```python
from build123d import *

# Parameters (mm, degrees)
SKETCH1_W           = 160
SKETCH1_H           = 28.575
BOSS_EXTRUDE1_DEPTH = 28.575
SKETCH3_W           = 147.3
SKETCH3_H           = 28.575
CUT_EXTRUDE3_DEPTH  = 19.05
SKETCH4_W           = 76.2
SKETCH4_H           = 8
BOSS_EXTRUDE2_DEPTH = 45.4
CUT_EXTRUDE8_DEPTH  = 124.871382326
SKETCH9_R           = 4.7625
BOSS_EXTRUDE4_DEPTH = 12.525
SKETCH10_R          = 4.7625
CUT_EXTRUDE10_DEPTH = 124.871382326
CUT_EXTRUDE11_START = -41.9
SKETCH2_OUTSIDE_W   = 111.689
SKETCH2_OUTSIDE_H   = 66.289
SKETCH2_OUTSIDE_R   = 14.2875
CUT_EXTRUDE11_DEPTH = 41.9
CUT_EXTRUDE13_START = -41.9
SKETCH13_OUTSIDE_W  = 111.689
SKETCH13_OUTSIDE_H  = 66.289
SKETCH13_OUTSIDE_R  = 14.2875
CUT_EXTRUDE13_DEPTH = 41.9
SKETCH14_R          = 11.1125
CUT_EXTRUDE14_DEPTH = 6.35
CUT_EXTRUDE15_START = -6.35
SKETCH15_R          = 11.1125
CUT_EXTRUDE15_DEPTH = 6.35


with BuildPart() as part:
    # Sketch1 → Boss-Extrude1 (new body)
    with BuildSketch(Plane(origin=(0, 0, 0), x_dir=(1, 0, 0), z_dir=(0, 1, 0))):
        with Locations((-20.782379652, -9.554800327)):
            Rectangle(SKETCH1_W, SKETCH1_H)
    extrude(amount=BOSS_EXTRUDE1_DEPTH)

    # Sketch3 → Cut-Extrude3 (cut)
    with BuildSketch(Plane(origin=(0, 28.575, 0), x_dir=(1, 0, 0), z_dir=(0, 1, 0))):
        with Locations((-20.782379652, -9.554800327)):
            Rectangle(SKETCH3_W, SKETCH3_H)
    extrude(amount=-CUT_EXTRUDE3_DEPTH, mode=Mode.SUBTRACT)

    # Sketch4 → Boss-Extrude2 (add)
    with BuildSketch(Plane.XY.offset(23.842300327)):
        with Locations((-20.782379652, 4.7625)):
            Rectangle(SKETCH4_W, SKETCH4_H)
    extrude(amount=BOSS_EXTRUDE2_DEPTH)

    # Sketch5 → Cut-Extrude8 (cut, through all)
    with BuildSketch(Plane(origin=(0, 8.7625, 0), x_dir=(1, 0, 0), z_dir=(0, 1, 0))):
        Polygon((-13.013921372, -46.075787503), (-13.013921372, -69.242300327), (17.317620348, -69.242300327), (17.317620348, -23.842300327), align=None)
        Polygon((-28.550837933, -69.242300327), (-28.550837933, -46.075787503), (-58.882379652, -23.842300327), (-58.882379652, -69.242300327), align=None)
    extrude(amount=-CUT_EXTRUDE8_DEPTH, mode=Mode.SUBTRACT)

    # Sketch9 → Boss-Extrude4 (add)
    with BuildSketch(Plane(origin=(0, 8.7625, 0), x_dir=(1, 0, 0), z_dir=(0, 1, 0))):
        with BuildLine():
            Line((-28.550837933, -46.075787503), (-28.550837933, -69.242300327))
            Line((-28.550837933, -69.242300327), (-13.013921372, -69.242300327))
            Line((-13.013921372, -69.242300327), (-13.013921372, -46.075787503))
            ThreePointArc((-13.013921372, -46.075787503), (-20.782379652, -32.954800327), (-28.550837933, -46.075787503))
        make_face()
        with Locations(Location((-20.782379652, -41.815004419, 0), (0, 0, 180))):
            Circle(SKETCH9_R, mode=Mode.SUBTRACT)
    extrude(amount=BOSS_EXTRUDE4_DEPTH)

    # Sketch10 → Cut-Extrude10 (cut, through all)
    with BuildSketch(Plane(origin=(0, 8.7625, 0), x_dir=(1, 0, 0), z_dir=(0, 1, 0))):
        with Locations(Location((-20.782379652, -41.815004419, 0), (0, 0, 180))):
            Circle(SKETCH10_R)
    extrude(amount=-CUT_EXTRUDE10_DEPTH, mode=Mode.SUBTRACT)

    # Sketch2 outside → Cut-Extrude11 (cut)
    with BuildSketch(Plane(origin=(59.217620348, 0, 0), x_dir=(0, 0, -1), z_dir=(1, 0, 0)).offset(CUT_EXTRUDE11_START)):
        with Locations((-32.2545, 14.2875)):
            Rectangle(SKETCH2_OUTSIDE_W, SKETCH2_OUTSIDE_H)
        with Locations((-9.554800327, 14.2875)):
            Circle(SKETCH2_OUTSIDE_R, mode=Mode.SUBTRACT)
    extrude(amount=CUT_EXTRUDE11_DEPTH, mode=Mode.SUBTRACT)

    # Sketch13 outside → Cut-Extrude13 (cut)
    with BuildSketch(Plane.ZY.offset(100.782379652).offset(CUT_EXTRUDE13_START)):
        with Locations((32.2545, 14.2875)):
            Rectangle(SKETCH13_OUTSIDE_W, SKETCH13_OUTSIDE_H)
        with Locations(Location((9.554800327, 14.2875, 0), (0, 0, 180))):
            Circle(SKETCH13_OUTSIDE_R, mode=Mode.SUBTRACT)
    extrude(amount=CUT_EXTRUDE13_DEPTH, mode=Mode.SUBTRACT)

    # Sketch14 → Cut-Extrude14 (cut)
    with BuildSketch(Plane(origin=(59.217620348, 0, 0), x_dir=(0, 0, -1), z_dir=(1, 0, 0))):
        with Locations((-9.554800327, 14.2875)):
            Circle(SKETCH14_R)
    extrude(amount=-CUT_EXTRUDE14_DEPTH, mode=Mode.SUBTRACT)

    # Sketch15 → Cut-Extrude15 (cut)
    with BuildSketch(Plane.ZY.offset(100.782379652).offset(CUT_EXTRUDE15_START)):
        with Locations(Location((9.554800327, 14.2875, 0), (0, 0, 180))):
            Circle(SKETCH15_R)
    extrude(amount=CUT_EXTRUDE15_DEPTH, mode=Mode.SUBTRACT)


solid = part.part
```
Here's how the part is built. I have some questions about the finished solid (model axes, mm). A direction names the side the tool comes from. Give positions to 0.01 mm unless a question says otherwise; leave off trailing zeros. Order: outer loops, then holes, each group sorted by start corner. A loop starts at its lowest first (then second) coordinate and runs counter-clockwise, first axis right, second up. Notation, with made-up numbers: M -12,-13.75 L 40,-13.75 A13 cw 40,-6.75 Z; hole C -31.5,73.25 d10. An arc over 180 degrees is marked long. Use a Markdown table: item, result. Add a question column.
1. Suppose I cut it at C-C (z = 15). List the corners of the cut face in (x, y) for me (3 decimals), and give its area (3 significant figures).
2. Suppose I cut it at D-D (y = 23.75). List the corners of the cut face in (x, z) for me.
3. Suppose I cut it at A-A (y = 16.25). List the corners of the cut face in (x, z) for me (1 decimal), and give its area (3 significant figures).
4. If we mould it in two halves opening along Y, with no side actions, what happens to faces 5 (the flat face through (-21, 21.288, 51)), 6 (the flat face through (-94.432, 7, 10)), 7 (the flat face through (-21, 0.763, 35)), 8 (the flat face through (-43.504, 4.818, 35.115))? For each: +Y half, -Y half, draft (parallel to the pull), parting line (faces both ways), or undercut.
5. For pin 1 Ø8 at (y, z) = (8, 6.5) entering from -X; pin 2 Ø8 at (y, z) = (7, 24.5) entering from +X; pin 3 Ø11 at (x, z) = (-34.5, 34) entering from +Y; pin 4 Ø14.5 at (x, z) = (-6.5, 8) entering from +Y (3 decimals), each with a flat end and sliding along its axis, tell me the tip position at first contact or that it passes through.
6. On a 3-axis mill with a long thin cutter (end or side, diameter ignored), from which of +Z, -Z, +X, -X, +Y, -Y can I reach the whole of each face in a straight line? I mean faces 1 (the cylindrical face through (-97.563, 10.95, -1.045)), 2 (the flat face through (-13.014, 11, 58)), 3 (the cylindrical face through (-20.53, 14.94, 32.96)), 4 (the flat face through (17.318, 3, -1)). Say none if no direction works.
7. I need wall thicknesses on probe 1 along X at (y, z) = (16, 42); probe 2 along X at (y, z) = (14.5, 54.5); probe 3 along X at (y, z) = (8.25, 13). Which ranges of each line are inside material? Lowest first, please. Write a range as from..to.
8. Suppose I cut it at B-B (x = -22.5). List the corners of the cut face in (y, z) for me (1 decimal), and give its area (3 significant figures).
Results list:
| question | item | result |
|---|---|---|
| 1 | outline | M -100.782,1.078 L -58.882,1.078 L -58.882,0 L 17.318,0 L 17.318,1.078 L 59.218,1.078 L 59.218,4.601 L 52.868,4.601 L 52.868,9.525 L -94.432,9.525 L -94.432,4.601 L -100.782,4.601 Z; M -100.782,23.974 L -94.432,23.974 L -94.432,27.497 L -100.782,27.497 Z; M 52.868,23.974 L 59.218,23.974 L 59.218,27.497 L 52.868,27.497 Z |
| 1 | area | 1,420 mm² |
| 2 | outline | M -100.78,-1.15 L -94.43,-1.15 L -94.43,3.73 L -100.78,3.73 Z; M -100.78,15.38 L -94.43,15.38 L -94.43,20.26 L -100.78,20.26 Z; M 52.87,-1.15 L 59.22,-1.15 L 59.22,3.73 L 52.87,3.73 Z; M 52.87,15.38 L 59.22,15.38 L 59.22,20.26 L 52.87,20.26 Z |
| 3 | outline | M -100.8,-4.6 L -94.4,-4.6 L -94.4,-1.4 L -100.8,-1.4 Z; M -100.8,20.5 L -94.4,20.5 L -94.4,23.7 L -100.8,23.7 Z; M -28.6,46.1 A8.9 ccw long -13,46.1 L -13,69.2 L -28.6,69.2 Z; M 52.9,-4.6 L 59.2,-4.6 L 59.2,-1.4 L 52.9,-1.4 Z; M 52.9,20.5 L 59.2,20.5 L 59.2,23.7 L 52.9,23.7 Z; hole C -20.8,41.8 d9.5 |
| 3 | area | 566 mm² |
| 4 | face 5 | +Y half |
| 4 | face 6 | undercut |
| 4 | face 7 | -Y half |
| 4 | face 8 | draft |
| 5 | pin 1 | stops at x = -94.43 |
| 5 | pin 2 | stops at x = 59.22 |
| 5 | pin 3 | stops at y = 8.76 |
| 5 | pin 4 | stops at y = 9.525 |
| 6 | face 1 | -X |
| 6 | face 2 | +Z, +X, +Y, -Y |
| 6 | face 3 | +Y |
| 6 | face 4 | -Z, +X, -Y |
| 7 | probe 1 | x = -29.64..-25.54, -16.02..-11.92 |
| 7 | probe 2 | x = -28.55..-13.01 |
| 7 | probe 3 | x = -94.43..52.87 |
| 8 | outline | M 0,-4.7 L 9.5,-4.7 L 9.5,23.8 L 8.8,23.8 L 8.8,33.1 L 21.3,33.1 L 21.3,37.4 L 0.8,37.4 L 0.8,23.8 L 0,23.8 Z; M 0.8,46.3 L 21.3,46.3 L 21.3,69.2 L 0.8,69.2 Z |
| 8 | area | 905 mm² |
